Can you work these out from the drawing? Everything is in mm from the part's minimum corner. A direction names the side the tool comes from. Round coordinates to 2 decimals unless told otherwise and drop trailing zeros. Order: outer loops, then holes, each group sorted by start corner. A loop starts at its lowest first (then second) coordinate and runs counter-clockwise, first axis right, second up. Notation, with made-up numbers: (-16.5, 19) - (22.5, 19) arc R18 ccw to (22.5, 33) - close; hole circle Ø10 at (47.25, 62.5). An arc over 180 degrees is marked (long way). Write item = value, one per line.
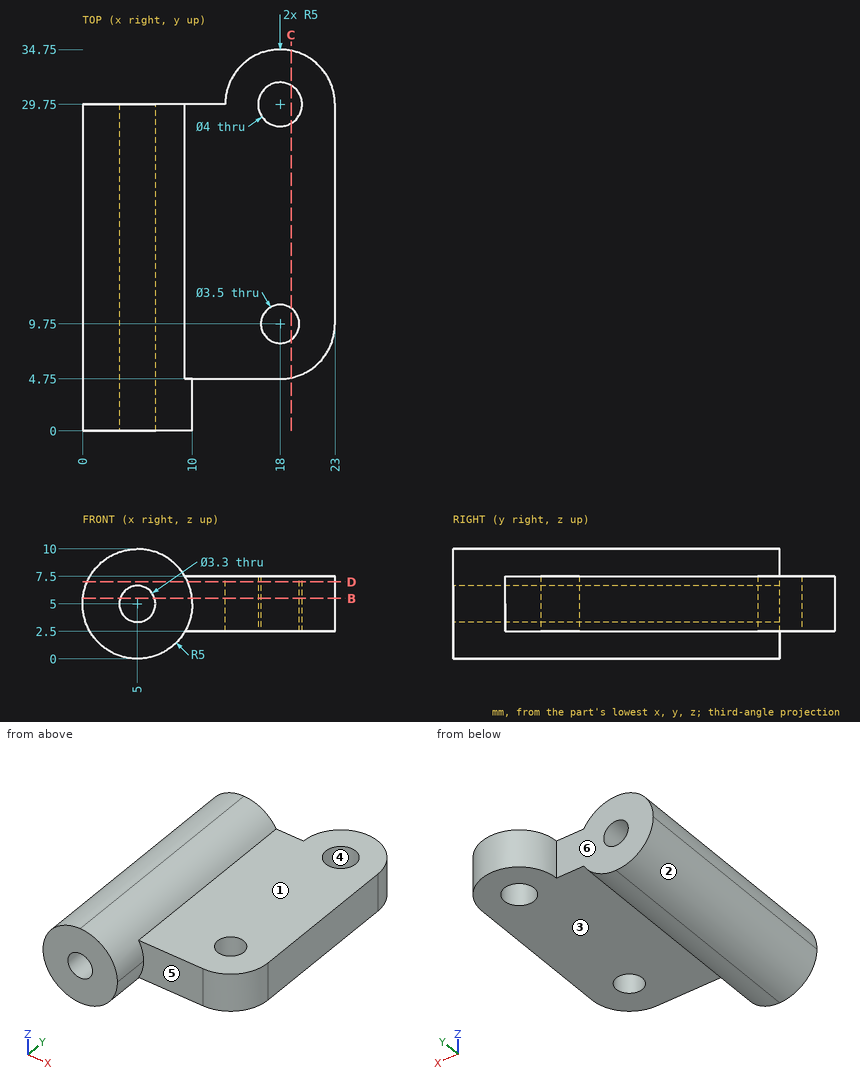
(1) If I drill on line 1 (Y direction, x = 18, z = 4.35); line 2 (Z direction, x = 6, y = 10); line 3 (Y direction, x = 2, z = 3.5), over which ranges is the centre line in solid material (lowest first)? Write a range as from..to.
Computed:
line_1 = 4.75..8, 11.5..27.75, 31.75..34.75
line_2 = 0.1..3.69, 6.31..9.9
line_3 = 0..29.75
(2) If we section it at C-C (x = 19): Write out the boundary of the cut face in (y, z), plus the area to 3 significant figures.
Computed:
outline = (4.85, 2.5) - (8.31, 2.5) - (8.31, 7.5) - (4.85, 7.5) - close; (11.19, 2.5) - (28.02, 2.5) - (28.02, 7.5) - (11.19, 7.5) - close; (31.48, 2.5) - (34.65, 2.5) - (34.65, 7.5) - (31.48, 7.5) - close
area = 117 mm^2
(3) On a 3-axis mill with a long thin cutter (end or side, diameter ignored), from which of +Z, -Z, +X, -X, +Y, -Y can I reach the whole of each face in a straight line? I mean the marked faces 1 and 2. Say none if no direction works.
Computed:
face_1 = +Z, +X, +Y, -Y
face_2 = -Z, -X, +Y, -Y
(4) If we section it at D-D (z = 7): Write out the boundary of the cut face in (x, y), plus the area to 3 significant figures.
Computed:
outline = (0.42, 0) - (9.58, 0) - (9.58, 4.75) - (18, 4.75) arc R5 ccw to (23, 9.75) - (23, 29.75) arc R5 ccw to (13, 29.75) - (0.42, 29.75) - close; hole circle Ø4 at (18, 29.75); hole circle Ø3.5 at (18, 9.75)
area = 620 mm^2
(5) Thinking about a two-plate mould opening in Y: for the marked faces 3, 4, 5 and 6, which applies, +Y half, -Y half, draft (parallel to the pull), parting line (faces both ways), or undercut?
Computed:
face_3 = draft
face_4 = undercut
face_5 = -Y half
face_6 = +Y half
(6) If we section it at B-B (z = 5.5): Write out the boundary of the cut face in (x, y).
Computed:
outline = (0.03, 0) - (3.43, 0) - (3.43, 29.75) - (0.03, 29.75) - close; (6.57, 0) - (9.97, 0) - (9.97, 4.75) - (18, 4.75) arc R5 ccw to (23, 9.75) - (23, 29.75) arc R5 ccw to (13, 29.75) - (6.57, 29.75) - close; hole circle Ø4 at (18, 29.75); hole circle Ø3.5 at (18, 9.75)
(7) Will these pins go through, and if not, where does the flat tip stop? P1, Ø4, axis at x = 11.5, z = 6, coming from the -Y side; P2, Ø4, axis at x = 19.5, y = 15.5, coming from the -Z side; P3, Ø1.5, axis at x = 10, y = 28.5, coming from the +Z side; P4, Ø8, axis at x = 15, y = 7, coming from the +Z side.
Computed:
P1 = 0
P2 = 2.5
P3 = 7.63
P4 = 7.5
